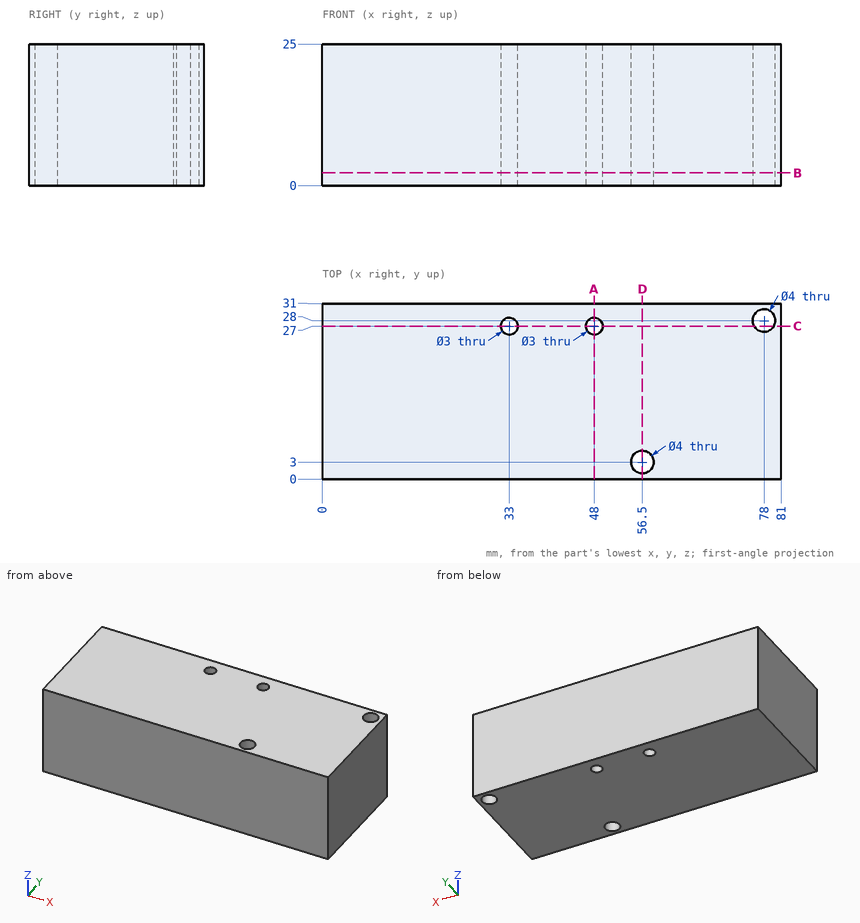
For this review, use the dimensioned drawing (mm, ordinates from the lowest corner) and the shaded views. Round coordinates to 2 decimals unless told otherwise and drop trailing zeros. Loops run counter-clockwise (first coordinate to the right, second up) from the corner with the lowest first, then second, coordinate; pieces in that order, holes last. Notation, with made-up numbers: M -32,17.25 L -23,17.25 A37 ccw -23,53.25 Z; hole C 27,5.5 d6. An arc over 180 degrees is marked long. Answer as CSV lines item,"result".
1. We need section B-B (z = 2.25). Give the boundary of the cut face in (x, y), plus the area to 3 significant figures.
Outcome:
outline,"M 0,0 L 81,0 L 81,31 L 0,31 Z; hole C 33,27 d3; hole C 48,27 d3; hole C 56.5,3 d4; hole C 78,28 d4"
area,"2,470 mm2"
2. We need section D-D (x = 56.5). Give the boundary of the cut face in (y, z).
Outcome:
outline,"M 0,0 L 1,0 L 1,25 L 0,25 Z; M 5,0 L 31,0 L 31,25 L 5,25 Z"
3. Insertion check: pin 1 Ø3.5 at (x, y) = (78, 28) entering from +Z. The pin has a flat end and moves straight along its axis. Give the tip position at first contact, or say it passes through.
Outcome:
pin 1,"passes through"
4. We need section C-C (y = 27). Give the boundary of the cut face in (x, z).
Outcome:
outline,"M 0,0 L 31.5,0 L 31.5,25 L 0,25 Z; M 34.5,0 L 46.5,0 L 46.5,25 L 34.5,25 Z; M 49.5,0 L 76.27,0 L 76.27,25 L 49.5,25 Z; M 79.73,0 L 81,0 L 81,25 L 79.73,25 Z"
5. To check wall thickness, follow L1, parallel to Y at x = 56.5, z = 8.5; L2, parallel to X at y = 28, z = 19.25; L3, parallel to X at y = 26.5, z = 16.75. State the ranges of each line that lie inside material, in increasing order. Write a range as [from, to].
Outcome:
L1,"y = [0, 1], [5, 31]"
L2,"x = [0, 31.88], [34.12, 46.88], [49.12, 76], [80, 81]"
L3,"x = [0, 31.59], [34.41, 46.59], [49.41, 76.68], [79.32, 81]"
6. We need section A-A (x = 48). Give the boundary of the cut face in (y, z), plus the area to 3 significant figures.
Outcome:
outline,"M 0,0 L 25.5,0 L 25.5,25 L 0,25 Z; M 28.5,0 L 31,0 L 31,25 L 28.5,25 Z"
area,"700 mm2"
